Geometry check sheet. Reference: the model listing, model coordinates, mm. A direction names the side the tool comes from. Give positions to 0.01 mm unless a question says otherwise; leave off trailing zeros. Loops run counter-clockwise (first coordinate to the right, second up) from the corner with the lowest first, then second, coordinate; pieces in that order, holes last. Notation, with made-up numbers: (-39, 20) -> (-35, 20) arc R12 cw to (-35, 43) -> close; hole circle Ø1 at (-40, -10.75). An arc over 180 degrees is marked (long way). Write item = value, one per line. Start each with the question number.
```python
from build123d import *

# Parameters (mm, degrees)
F0_W     = 118.7196
F0_H     = 38.1
F1_DEPTH = 25.4
F2_W     = 25.4
F2_H     = 31.75
F3_DEPTH = 12.7
F4_W     = 12.7
F4_H     = 3.175
F5_DEPTH = 12.7
F6_W     = 12.7
F6_H     = 3.175
F7_DEPTH = 12.7
F8_R     = 3.175
F9_DEPTH = 25.4


with BuildPart() as f1:
    # F0 (on Top) → F1 (new body)
    with BuildSketch(Plane.XY):
        Rectangle(F0_W, F0_H)
    extrude(amount=F1_DEPTH)

    # F2 (on face) → F3 (join)
    with BuildSketch(Plane(origin=(0, 0, 0), x_dir=(1, 0, 0), z_dir=(0, 0, -1))):
        with Locations((-33.9598, 0)):
            Rectangle(F2_W, F2_H)
        with Locations((33.9598, 0)):
            Rectangle(F2_W, F2_H)
    extrude(amount=F3_DEPTH)

    # F4 (on face) → F5 (join)
    with BuildSketch(Plane(origin=(0, 0, -12.7), x_dir=(1, 0, 0), z_dir=(0, 0, -1))):
        with Locations((-33.9598, 14.2875)):
            Rectangle(F4_W, F4_H)
        with Locations((-33.9598, -14.2875)):
            Rectangle(F4_W, F4_H)
    extrude(amount=F5_DEPTH)

    # F6 (on face) → F7 (join)
    with BuildSketch(Plane(origin=(0, 0, -12.7), x_dir=(1, 0, 0), z_dir=(0, 0, -1))):
        with Locations((33.9598, 14.2875)):
            Rectangle(F6_W, F6_H)
        with Locations((33.9598, -14.2875)):
            Rectangle(F6_W, F6_H)
    extrude(amount=F7_DEPTH)

    # F8 (on face) → F9 (join)
    with BuildSketch(Plane.XY.offset(25.4)):
        Circle(F8_R)
    extrude(amount=F9_DEPTH)


solid = f1.part
```
1) Section check B-B (x = 0). Enter the section's corners in (y, z) (3 decimals).
2) Section check D-D (z = 35). Enter the section's corners in (x, y) (3 decimals), plus the area to 3 significant figures.
3) Section check A-A (z = -19). Enter the section's corners in (x, y) (3 decimals).
4) Thickness scan on line 1 (X direction, y = -13, z = -15.5); line 2 (Y direction, x = -28, z = -14) (3 decimals); line 3 (Y direction, x = 29, z = -2) (3 decimals). Record the ranges inside material, lowest first.
5) Depth check by flat-ended pin: pin 1 Ø1 at (y, z) = (14.5, -16.5) entering from +X; pin 2 Ø1 at (x, y) = (3.5, -10.5) entering from +Z; pin 3 Ø10 at (x, z) = (-31.5, -17.5) entering from -Y (3 decimals). Enter the tip coordinate at first touch or a pass-through.
6) Draft check along X on faces 6 (the flat face through (-27.61, -14, -19)), 7 (the flat face through (46.66, 0, -6)), 8 (the cylindrical face through (-0.69, -3.1, 37.92)), 9 (the flat face through (-34, -12.7, -19)). Enter one of: released by +X, released by -X, zero draft, split by the parting line, or undercut.
7) Section check C-C (y = 6). Enter the section's corners in (x, z).
8) Tool access check on faces 1 (the flat face through (34, 15.875, -10)), 2 (the flat face through (21.26, 0, -6)), 3 (the flat face through (-34, 14, -25.4)), 4 (the flat face through (34, -15.875, -10)), 5 (the flat face through (34, -12.7, -19)). Record the directions out of +Z, -Z, +X, -X, +Y, -Y that give a thin tool (end or side, any length) a straight path to the whole face; none if there is none.
Check result:
q1.outline = (-19.05, 0) -> (19.05, 0) -> (19.05, 25.4) -> (3.175, 25.4) -> (3.175, 50.8) -> (-3.175, 50.8) -> (-3.175, 25.4) -> (-19.05, 25.4) -> close
q2.outline = circle Ø6.35 at (0, 0)
q2.area = 31.7 mm2
q3.outline = (-40.31, -15.875) -> (-27.61, -15.875) -> (-27.61, -12.7) -> (-40.31, -12.7) -> close; (-40.31, 12.7) -> (-27.61, 12.7) -> (-27.61, 15.875) -> (-40.31, 15.875) -> close; (27.61, -15.875) -> (40.31, -15.875) -> (40.31, -12.7) -> (27.61, -12.7) -> close; (27.61, 12.7) -> (40.31, 12.7) -> (40.31, 15.875) -> (27.61, 15.875) -> close
q4.line_1 = -40.31 to -27.61, 27.61 to 40.31
q4.line_2 = -15.875 to -12.7, 12.7 to 15.875
q4.line_3 = -15.875 to 15.875
q5.pin_1 = 40.31
q5.pin_2 = 25.4
q5.pin_3 = -15.875
q6.face_6 = undercut
q6.face_7 = released by +X
q6.face_8 = split by the parting line
q6.face_9 = zero draft
q7.outline = (-59.36, 0) -> (-46.66, 0) -> (-46.66, -12.7) -> (-21.26, -12.7) -> (-21.26, 0) -> (21.26, 0) -> (21.26, -12.7) -> (46.66, -12.7) -> (46.66, 0) -> (59.36, 0) -> (59.36, 25.4) -> (-59.36, 25.4) -> close
q8.face_1 = -Z, +X, -X, +Y
q8.face_2 = -Z, +Y, -Y
q8.face_3 = -Z, +X, -X, +Y, -Y
q8.face_4 = -Z, +X, -X, -Y
q8.face_5 = -Z, +X, -X
